Source: CAD feature listing. Evaluate the final solid. Frame: model axes, mm. Face numbers are marked on the shaded views. A direction names the side the tool comes from. Coordinates: 2 decimals unless noted, no trailing zeros. Write each loop counter-clockwise with the first axis right and the second up, starting at its lowest first coordinate (ties: lowest second). Pieces come first, ordered by that corner, then holes. Notation, with made-up numbers: M -19.5,23 L 16.5,23 A27 cw 16.5,54 Z; hole C 21.25,-38.75 d5. An arc over 180 degrees is marked long. One line per item, written item: value. Start each with the question number.
Item 1: Cut plane C-C, the plane z = 7.5. Output: boundary loops of the cut face in (x, y), then the cut area to 3 significant figures.
Item 2: Ray query, L1, parallel to Y at x = 37.5, z = 11.25; L2, parallel to X at y = 14.5, z = 0.85; L3, parallel to X at y = 71.5, z = 1.95. Return the intervals inside material, ascending. Write a range as from..to.
Item 3: Pin query (flat end, axial travel): P1, Ø6, axis at y = 79.5, z = 13, coming from the -X side; P2, Ø2, axis at x = 14.5, y = 79.5, coming from the +Z side; P3, Ø4.5, axis at x = 24, y = 90.5, coming from the -Z side. Return the tip coordinate at first contact, or that it passes through.
Item 4: Mould query, pull axis X, two halves, no side actions, for the marked faces 4, 5, 6 and 7. Classes: released by +X, released by -X, zero draft, split by the parting line, or undercut.
Item 5: Cut plane A-A, the plane x = 52.5. Output: boundary loops of the cut face in (y, z), then the cut area to 3 significant figures.
Item 6: Cut plane D-D, the plane x = 24. State how many separate pieces and enclosed holes the cut face has, then the cut area to 3 significant figures.
Item 7: Cut plane B-B, the plane y = 14.5. Output: boundary loops of the cut face in (x, z), then the cut area to 3 significant figures.
Item 8: Set-up query: the marked faces 1, 2 and 3. Return all of +Z, -Z, +X, -X, +Y, -Y with unobstructed straight access to the full face (end or side cutting, diameter ignored); none if empty.
```python
from build123d import *

# Parameters (mm, degrees)
PAD001_DEPTH    = 17
SKETCH003_W     = 59
SKETCH003_H     = 97
POCKET001_DEPTH = 14
SKETCH004_R     = 3
POCKET002_DEPTH = 1
SKETCH005_R     = 1.3
POCKET003_DEPTH = 3
SKETCH006_R     = 2.5
POCKET004_DEPTH = 1
FILLET001_R     = 7
FILLET002_R     = 2
FILLET003_R     = 2
SKETCH007_R     = 28.5
POCKET005_DEPTH = 3
SKETCH012_W     = 25
SKETCH012_H     = 2
POCKET007_DEPTH = 3.5
POCKET008_DEPTH = 6


with BuildPart() as part:
    # Sketch002 → Pad001 (new body)
    with BuildSketch(Plane.XY):
        with BuildLine():
            Line((0, 0), (69, 0))
            Line((69, 0), (69, 107))
            Line((69, 107), (0, 107))
            Line((0, 107), (0, 76.215633))
            ThreePointArc((0, 76.215633), (-12, 53.5), (0, 30.784367))
            Line((0, 0), (0, 30.784367))
        make_face()
    extrude(amount=PAD001_DEPTH)

    # Sketch003 (on Face8 of Pad001) → Pocket001 (cut)
    with BuildSketch(Plane.XY.offset(17)):
        with Locations((34.5, 53.5)):
            Rectangle(SKETCH003_W, SKETCH003_H)
    extrude(amount=-POCKET001_DEPTH, mode=Mode.SUBTRACT)

    # Sketch004 (on Face4 of Pocket001) → Pocket002 (cut)
    with BuildSketch(Plane(origin=(0, 0, 0), x_dir=(1, 0, 0), z_dir=(0, 0, -1))):
        with Locations((6, -6)):
            Circle(SKETCH004_R)
        with Locations((63, -6)):
            Circle(SKETCH004_R)
        with Locations((6, -101)):
            Circle(SKETCH004_R)
        with Locations((63, -101)):
            Circle(SKETCH004_R)
        with Locations((6, -37.666667)):
            Circle(SKETCH004_R)
        with Locations((6, -69.333333)):
            Circle(SKETCH004_R)
        with Locations((63, -37.666667)):
            Circle(SKETCH004_R)
        with Locations((63, -69.333333)):
            Circle(SKETCH004_R)
        with Locations((-6.5, -53.5)):
            Circle(SKETCH004_R)
    extrude(amount=-POCKET002_DEPTH, mode=Mode.SUBTRACT)

    # Sketch005 (on Face31 of Pocket002) → Pocket003 (cut)
    with BuildSketch(Plane.XY.offset(3)):
        with Locations((24, 14.5)):
            Circle(SKETCH005_R)
        with Locations((43, 14.5)):
            Circle(SKETCH005_R)
        with Locations((52.5, 24)):
            Circle(SKETCH005_R)
        with Locations((43, 33.5)):
            Circle(SKETCH005_R)
        with Locations((24, 33.5)):
            Circle(SKETCH005_R)
        with Locations((24.000052, 71.5)):
            Circle(SKETCH005_R)
        with Locations((43, 71.5)):
            Circle(SKETCH005_R)
        with Locations((43, 90.5)):
            Circle(SKETCH005_R)
        with Locations((24, 90.5)):
            Circle(SKETCH005_R)
        with Locations((52.5, 81)):
            Circle(SKETCH005_R)
    extrude(amount=-POCKET003_DEPTH, mode=Mode.SUBTRACT)

    # Sketch006 (on Face4 of Pocket003) → Pocket004 (cut)
    with BuildSketch(Plane(origin=(0, 0, 0), x_dir=(1, 0, 0), z_dir=(0, 0, -1))):
        with Locations((24, -14.5)):
            Circle(SKETCH006_R)
        with Locations((43, -14.5)):
            Circle(SKETCH006_R)
        with Locations((52.5, -24)):
            Circle(SKETCH006_R)
        with Locations((43, -33.5)):
            Circle(SKETCH006_R)
        with Locations((24, -33.5)):
            Circle(SKETCH006_R)
        with Locations((52.5, -81)):
            Circle(SKETCH006_R)
        with Locations((43, -71.5)):
            Circle(SKETCH006_R)
        with Locations((24.000052, -71.5)):
            Circle(SKETCH006_R)
        with Locations((24, -90.5)):
            Circle(SKETCH006_R)
        with Locations((43, -90.5)):
            Circle(SKETCH006_R)
    extrude(amount=-POCKET004_DEPTH, mode=Mode.SUBTRACT)

    # Fillet001
    fillet001_edges = [part.edges().sort_by_distance(p)[0] for p in [
        (69, 0, 8.5),
        (0, 0, 8.5),
        (69, 107, 8.5),
        (0, 107, 8.5),
    ]]
    fillet(fillet001_edges, radius=FILLET001_R)

    # Fillet002
    fillet002_edges = [part.edges().sort_by_distance(p)[0] for p in [
        (64, 102, 10),
        (64, 5, 10),
        (5, 5, 10),
        (5, 102, 10),
    ]]
    fillet(fillet002_edges, radius=FILLET002_R)

    # Fillet003
    fillet003_edges = [part.edges().sort_by_distance(p)[0] for p in [
        (34.5, 0, 0),
        (-12, 53.5, 0),
        (0, 18.892183, 17),
    ]]
    fillet(fillet003_edges, radius=FILLET003_R)

    # Sketch007 (on Face1 of Fillet003) → Pocket005 (cut)
    with BuildSketch(Plane.XY.offset(17)):
        with Locations((15.5, 53.5)):
            Circle(SKETCH007_R)
    extrude(amount=-POCKET005_DEPTH, mode=Mode.SUBTRACT)

    # Sketch012 (on Face16 of Pocket005) → Pocket007 (cut)
    with BuildSketch(Plane(origin=(64, 0, 0), x_dir=(0, -1, 0), z_dir=(-1, 0, 0))):
        with Locations((-53.5, 10)):
            Rectangle(SKETCH012_W, SKETCH012_H)
    extrude(amount=-POCKET007_DEPTH, mode=Mode.SUBTRACT)

    # Sketch013 (on Face16 of Pocket007) → Pocket008 (cut)
    with BuildSketch(Plane(origin=(64, 0, 0), x_dir=(0, -1, 0), z_dir=(-1, 0, 0))):
        with BuildLine():
            Line((-56.5, 9.5), (-50.5, 9.5))
            ThreePointArc((-50.5, 5.5), (-48.5, 7.5), (-50.5, 9.5))
            Line((-56.5, 5.5), (-50.5, 5.5))
            ThreePointArc((-56.5, 9.5), (-58.5, 7.5), (-56.5, 5.5))
        make_face()
    extrude(amount=-POCKET008_DEPTH, mode=Mode.SUBTRACT)


solid = part.part
```
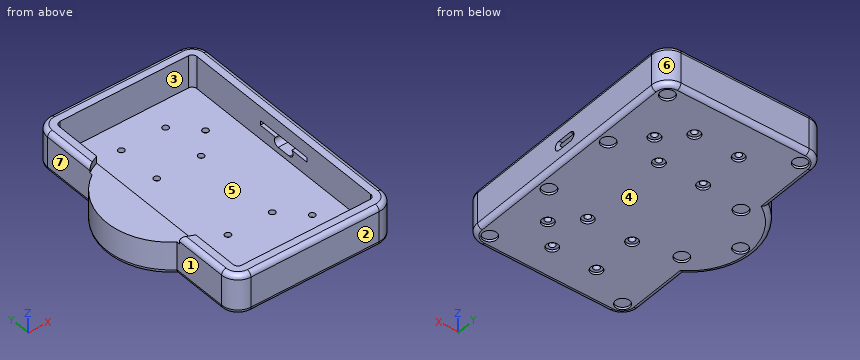
From the geometry:
1. outline: M 0,7 A7 ccw 7,0 L 62,0 A7 ccw 69,7 L 69,48.5 L 64,48.5 L 64,7 A2 cw 62,5 L 7,5 A2 cw 5,7 L 5,100 A2 cw 7,102 L 62,102 A2 cw 64,100 L 64,58.5 L 69,58.5 L 69,100 A7 ccw 62,107 L 7,107 A7 ccw 0,100 L 0,76.22 A27.5 ccw 0,30.78 Z
1. area: 1,950 mm²
2. L1: y = 0..5, 102..107
2. L2: x = 0.36..21.5, 26.5..40.5, 45.5..68.64
2. L3: x = -5.29..22.7, 25.3..41.7, 44.3..69
3. P1: stops at x = 0
3. P2: stops at z = 3
3. P3: stops at z = 1
4. face 4: zero draft
4. face 5: undercut
4. face 6: released by +X
4. face 7: released by -X
5. outline: M 0,2 A2 ccw 2,0 L 21.5,0 L 21.5,1 L 22.7,1 L 22.7,3 L 5,3 L 5,17 L 2,17 A2 ccw 0,15 Z; M 25.3,1 L 26.5,1 L 26.5,0 L 78.5,0 L 78.5,1 L 79.7,1 L 79.7,3 L 25.3,3 Z; M 82.3,1 L 83.5,1 L 83.5,0 L 105,0 A2 ccw 107,2 L 107,15 A2 ccw 105,17 L 102,17 L 102,3 L 82.3,3 Z
5. area: 437 mm²
6. separate pieces: 5
6. enclosed holes: 0
6. area: 417 mm²
7. outline: M 0,2 A2 ccw 2,0 L 21.5,0 L 21.5,1 L 22.7,1 L 22.7,3 L 5,3 L 5,17 L 2,17 A2 ccw 0,15 Z; M 25.3,1 L 26.5,1 L 26.5,0 L 40.5,0 L 40.5,1 L 41.7,1 L 41.7,3 L 25.3,3 Z; M 44.3,1 L 45.5,1 L 45.5,0 L 67,0 A2 ccw 69,2 L 69,15 A2 ccw 67,17 L 64,17 L 64,3 L 44.3,3 Z
7. area: 323 mm²
8. face 1: +Z, -Z, -X, -Y
8. face 2: +Z, -Z, +X, -X, -Y
8. face 3: +Z
